Source: three-view drawing plus pictorial views. Frame: mm from the lowest corner of the part. Give positions to 0.01 mm unless a question says otherwise; leave off trailing zeros. Order: outer loops, then holes, each group sorted by start corner. A loop starts at its lowest first (then second) coordinate and runs counter-clockwise, first axis right, second up. Notation, with made-up numbers: M 22.25,-13 L 41.25,-13 A15 cw 41.25,-7 Z; hole C -31,16 d8. An arc over 180 degrees is marked long. Use CSV: the item, a comma, the result in double quotes.
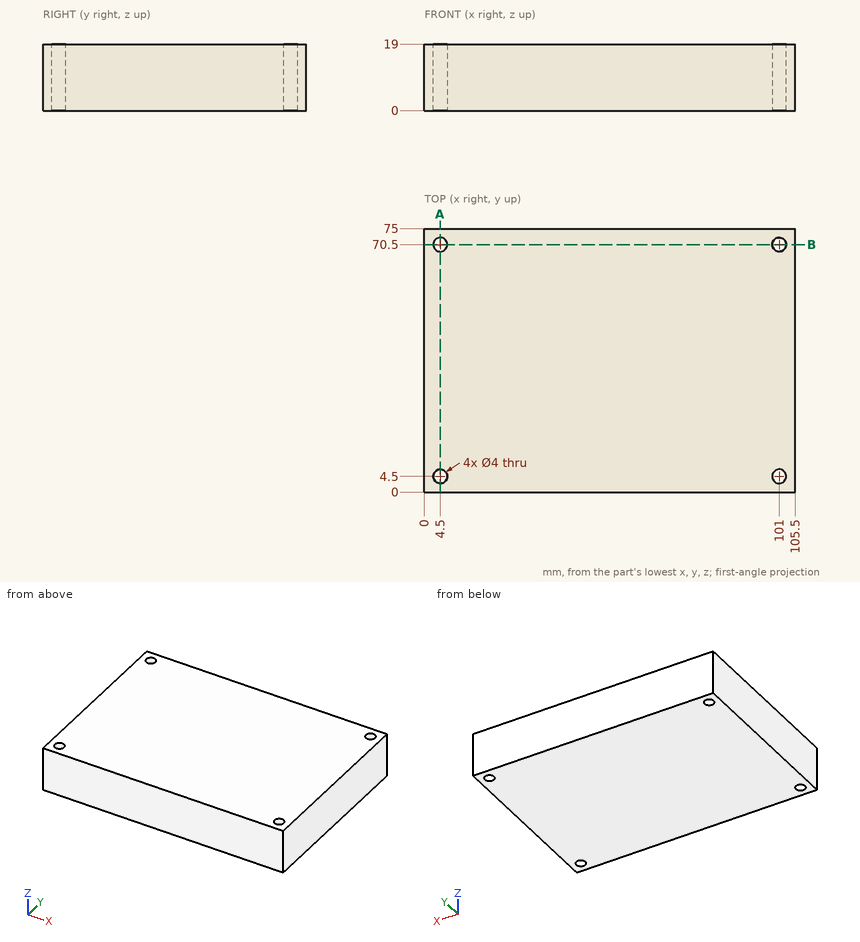
1. Pin query (flat end, axial travel): pin 1 Ø3 at (x, y) = (101, 4.5) entering from +Z. Return the tip coordinate at first contact, or that it passes through.
Answer:
pin 1,"through"
2. Line query: line 1 (Y direction, x = 4.5, z = 5.5); line 2 (X direction, y = 70.5, z = 8.5). Output: solid intervals per line, ascending.
Answer:
line 1,"0 to 2.5, 6.5 to 68.5, 72.5 to 75"
line 2,"0 to 2.5, 6.5 to 99, 103 to 105.5"
3. Section A-A, the plane x = 4.5. Return the cut outline in (y, z).
Answer:
outline,"M 0,0 L 2.5,0 L 2.5,19 L 0,19 Z; M 6.5,0 L 68.5,0 L 68.5,19 L 6.5,19 Z; M 72.5,0 L 75,0 L 75,19 L 72.5,19 Z"
4. Section B-B, the plane y = 70.5. Return the cut outline in (x, z).
Answer:
outline,"M 0,0 L 2.5,0 L 2.5,19 L 0,19 Z; M 6.5,0 L 99,0 L 99,19 L 6.5,19 Z; M 103,0 L 105.5,0 L 105.5,19 L 103,19 Z"
